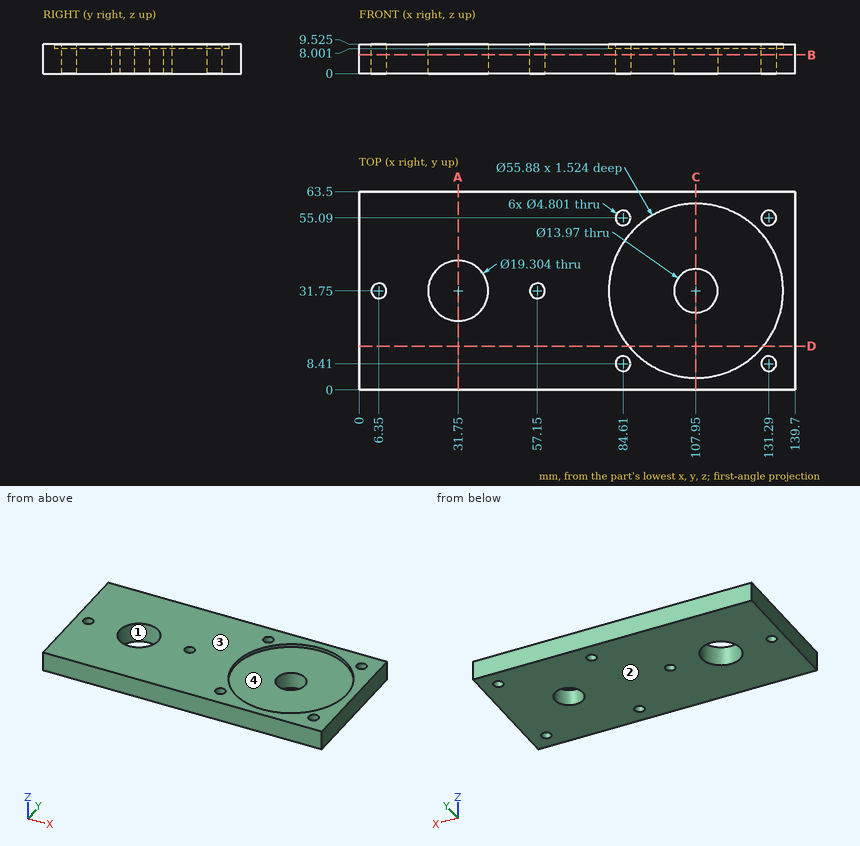
Geometry check sheet. Reference: drawing and pictorial views, mm from the part's lowest x, y, z. A direction names the side the tool comes from. Round coordinates to 2 decimals unless told otherwise and drop trailing zeros. Order: outer loops, then holes, each group sorted by start corner. A loop starts at its lowest first (then second) coordinate and runs counter-clockwise, first axis right, second up. Notation, with made-up numbers: (35, 77) -> (43, 77) arc R25 ccw to (43, 116) -> close; hole circle Ø2 at (-19, -21). An arc over 180 degrees is marked (long way). One line per item, written item: value. Start each with the question number.
Q1. Gauge pin test, flat ends, axial feed: pin 1 Ø4.5 at (x, y) = (6.35, 31.75) entering from -Z; pin 2 Ø6 at (x, y) = (131.29, 55.09) entering from +Z (3 decimals); pin 3 Ø1.5 at (x, y) = (110, 44) entering from +Z. Record the tip position at first contact, or that the pin passes through.
Q2. Cross-section at A-A (x = 31.75). Record the boundary of the cut face in (y, z) (1 decimal), and give its area (3 significant figures).
Q3. Cross-section at D-D (y = 14). Record the boundary of the cut face in (x, z) (1 decimal), and give its area (4 significant figures).
Q4. Cross-section at B-B (z = 6). Give the number of separate pieces and of enclosed holes in the cut face, and give its area (3 significant figures).
Q5. Mould release check, pull along X, two halves, no side actions. Record for the marked faces 1 and 2: pulls with the +X half, pulls with the -X half, needs draft (parallel to the pull), parting line crosses it, or undercut.
Q6. Set-up check for the marked faces 3 and 4: record each of +Z, -Z, +X, -X, +Y, -Y from which the full face is reachable in a straight line by a thin tool's end or side.
Q7. Thickness scan on line 1 (Y direction, x = 31.75, z = 4); line 2 (X direction, y = 54.5, z = 7); line 3 (X direction, y = 28, z = 1) (1 decimal). Record the ranges inside material, lowest first.
Q8. Cross-section at C-C (x = 107.95). Record the boundary of the cut face in (y, z) (1 decimal), and give its area (3 significant figures).
Completed:
1. pin 1: passes through
1. pin 2: stops at z = 9.525
1. pin 3: stops at z = 8
2. outline: (0, 0) -> (22.1, 0) -> (22.1, 9.5) -> (0, 9.5) -> close; (41.4, 0) -> (63.5, 0) -> (63.5, 9.5) -> (41.4, 9.5) -> close
2. area: 421 mm²
3. outline: (0, 0) -> (139.7, 0) -> (139.7, 9.5) -> (129.5, 9.5) -> (129.5, 8) -> (86.4, 8) -> (86.4, 9.5) -> (0, 9.5) -> close
3. area: 1,265 mm²
4. separate pieces: 1
4. enclosed holes: 8
4. area: 8,320 mm²
5. face 1: undercut
5. face 2: needs draft
6. face 3: +Z, +X, -X, +Y, -Y
6. face 4: +Z
7. line 1: y = 0 to 22.1, 41.4 to 63.5
7. line 2: x = 0 to 82.28, 86.94 to 128.96, 133.62 to 139.7
7. line 3: x = 0 to 22.9, 40.6 to 102.1, 113.8 to 139.7
8. outline: (0, 0) -> (24.8, 0) -> (24.8, 8) -> (3.8, 8) -> (3.8, 9.5) -> (0, 9.5) -> close; (38.7, 0) -> (63.5, 0) -> (63.5, 9.5) -> (59.7, 9.5) -> (59.7, 8) -> (38.7, 8) -> close
8. area: 408 mm²
